The listing builds one solid part. Answer for the finished solid, in the listing's coordinates (mm). A direction names the side the tool comes from. Coordinates: 2 decimals unless noted, no trailing zeros. Order: outer loops, then holes, each group sorted by start corner. A loop starts at its lowest first (then second) coordinate and runs counter-clockwise, first axis right, second up. Notation, with made-up numbers: (71, 25) - (91, 25) arc R31 cw to (91, 49) - close; hole circle Ø9 at (0, 41). An arc over 180 degrees is marked (long way). Use one line per item in the form item = value. Start each with the question number.
Item 1: Each of these flat-tipped pins is pushed along its axis until it touches: pin 1 Ø1.5 at (y, z) = (12.5, 4) entering from -X; pin 2 Ø6 at (y, z) = (11.5, 8) entering from -X; pin 3 Ø5.5 at (x, y) = (37.5, 13.5) entering from +Z. Where does it stop, or does it pass through?
Item 2: Section D-D, the plane z = -20 is taken. Write down the section's boundary in (x, y).
Item 3: Section B-B, the plane z = 0 is taken. Write down the section's boundary in (x, y).
Item 4: A tool of negligible diameter and unlimited length cuts with its end or side. For faces 1 (the flat face through (32.5, 12, 5)), 2 (the flat face through (0, 9.7, 0)), 3 (the flat face through (47.5, 12, -5)), from which of +Z, -Z, +X, -X, +Y, -Y can it reach the whole face along a straight path? Write none if from no direction.
Item 5: Consider line 1 along Z through (x, y) = (37, 13); line 2 along Y through (x, z) = (8.5, 14.5); line 3 along Y through (x, z) = (61.5, 5.5). Determine where each line is inside the solid, lowest interval first. Write a range as [from, to].
Item 6: Section A-A, the plane y = 13.5 is taken. Write down the section's boundary in (x, z).
Item 7: Section C-C, the plane y = 7.25 is taken. Write down the section's boundary in (x, z).
Item 8: The mould has two halves that part along Z. Classify faces 4 (the cylindrical face through (64.994, 4.93, -0.55)), 5 (the flat face through (40, 15, -5)), 6 (the flat face through (40, 12, -2.1)): released by +Z, released by -Z, zero draft, split by the parting line, or undercut.
from build123d import *

# Parameters (mm, degrees)
EXTRUDE_1_DEPTH     = 10
CUT_EXTRUDE_START   = -5
SKETCH_2_R          = 25
CUT_EXTRUDE_1_DEPTH = 5
SKETCH_3_R          = 2.5
EXTRUDE_2_DEPTH     = 4.7
SKETCH_4_W          = 15
SKETCH_4_H          = 6
EXTRUDE_3_DEPTH     = 5


with BuildPart() as part:
    # 草圖1 → 填料-伸長1 (new body)
    with BuildSketch(Plane(origin=(0, 0, 0), x_dir=(1, 0, 0), z_dir=(0, 1, 0))):
        with BuildLine():
            Line((0, 25), (40, 25))
            ThreePointArc((40, 25), (65, 0), (40, -25))
            Line((40, -25), (0, -25))
            ThreePointArc((0, -25), (-25, 0), (0, 25))
        make_face()
    extrude(amount=EXTRUDE_1_DEPTH)

    # 草圖2 → 除料-伸長1 (cut)
    with BuildSketch(Plane(origin=(0, 10, 0), x_dir=(1, 0, 0), z_dir=(0, 1, 0)).offset(CUT_EXTRUDE_START)):
        Circle(SKETCH_2_R)
    extrude(amount=CUT_EXTRUDE_1_DEPTH, mode=Mode.SUBTRACT)

    # 草圖3 → 填料-伸長2 (add)
    with BuildSketch(Plane(origin=(0, 5, 0), x_dir=(1, 0, 0), z_dir=(0, 1, 0))):
        with Locations(Location((0, 0, 0), (0, 0, 270))):
            Circle(SKETCH_3_R)
    extrude(amount=EXTRUDE_2_DEPTH)

    # 草圖4 → 填料-伸長3 (add)
    with BuildSketch(Plane(origin=(0, 10, 0), x_dir=(1, 0, 0), z_dir=(0, 1, 0))):
        with Locations((40, 5.1)):
            Rectangle(SKETCH_4_W, SKETCH_4_H)
        with Locations((40, -5.1)):
            Rectangle(SKETCH_4_W, SKETCH_4_H)
    extrude(amount=EXTRUDE_3_DEPTH)


solid = part.part
Response:
q1.pin_1 = 32.5
q1.pin_2 = 22.64
q1.pin_3 = 8.1
q2.outline = (-15, 0) - (55, 0) - (55, 10) - (15, 10) - (15, 5) - (-15, 5) - close
q3.outline = (-25, 0) - (65, 0) - (65, 10) - (25, 10) - (25, 5) - (2.5, 5) - (2.5, 9.7) - (-2.5, 9.7) - (-2.5, 5) - (-25, 5) - close
q4.face_1 = +Z, -Z, -X, +Y
q4.face_2 = -X, +Y
q4.face_3 = +Z, -Z, +X, +Y
q5.line_1 = [-8.1, -2.1], [2.1, 8.1]
q5.line_2 = [0, 5]
q5.line_3 = [0, 10]
q6.outline = (32.5, -8.1) - (47.5, -8.1) - (47.5, -2.1) - (32.5, -2.1) - close; (32.5, 2.1) - (47.5, 2.1) - (47.5, 8.1) - (32.5, 8.1) - close
q7.outline = circle Ø5 at (0, 0); (0, -25) - (40, -25) arc R25 ccw to (40, 25) - (0, 25) arc R25 cw to start
q8.face_4 = split by the parting line
q8.face_5 = zero draft
q8.face_6 = undercut
